Work out the finished part from the listing and answer in its coordinate system (mm). Face numbers are marked on the shaded views. Coordinates: 2 decimals unless noted, no trailing zeros. Write each loop counter-clockwise with the first axis right and the second up, starting at its lowest first coordinate (ties: lowest second). Pieces come first, ordered by that corner, then holes. Notation, with made-up numbers: (-38, 69.25) - (-27, 69.25) arc R34 cw to (-27, 101.25) - close; hole circle Ø8 at (11, 52). An arc over 180 degrees is marked (long way). Use CSV: the item, a comma, the result in double quotes. Start each with the question number.
from build123d import *

# Parameters (mm, degrees)
SKETCH1_W             = 48.6918
SKETCH1_H             = 39.1668
SKETCH1_R             = 4.7625
SKETCH1_R_2           = 3.175
BOSS_EXTRUDE1_DEPTH   = 7.62
CHAMFER1_SIZE         = 3.175
SKETCH3_W             = 39.1668
SKETCH3_H             = 29.6418
CUT_EXTRUDE2_DEPTH    = 1.27
F_4_CLEARANCE_HOLE1_D = 3.048
SKETCH7_R             = 4.415840843
SKETCH7_R_2           = 3.175
SKETCH7_R_3           = 1.5875
BOSS_EXTRUDE2_DEPTH   = 1.27
SKETCH15_R            = 6.0325
BOSS_EXTRUDE7_DEPTH   = 7.62
FILLET3_R             = 6.985
FILLET4_R             = 0.508


with BuildPart() as part:
    # Sketch1 → Boss-Extrude1 (new body)
    with BuildSketch(Plane.YZ):
        with Locations((-3.96875, 0)):
            Rectangle(SKETCH1_W, SKETCH1_H)
        with Locations(Location((-8.73125, 0, 0), (0, 0, 90))):
            Circle(SKETCH1_R, mode=Mode.SUBTRACT)
        with Locations(Location((8.73125, 0, 0), (0, 0, 90))):
            Circle(SKETCH1_R_2, mode=Mode.SUBTRACT)
    extrude(amount=BOSS_EXTRUDE1_DEPTH)

    # Chamfer1
    chamfer1_edges = [part.edges().sort_by_distance(p)[0] for p in [
        (3.81, 20.37715, -19.5834),
        (3.81, -28.31465, -19.5834),
        (3.81, -28.31465, 19.5834),
        (3.81, 20.37715, 19.5834),
    ]]
    chamfer(chamfer1_edges, length=CHAMFER1_SIZE)

    # Sketch3 → Cut-Extrude2 (cut)
    with BuildSketch(Plane(origin=(0, 0, 0), x_dir=(0, -1, 0), z_dir=(-1, 0, 0))):
        Polygon((-18.254252448, -22.1234), (26.191752448, -22.1234), (30.85465, -17.460502448), (30.85465, 17.460502448), (26.191752448, 22.1234), (-18.254252448, 22.1234), (-22.91715, 17.460502448), (-22.91715, -17.460502448), align=None)
        with Locations((3.96875, 0)):
            Rectangle(SKETCH3_W, SKETCH3_H, mode=Mode.SUBTRACT)
    extrude(amount=-CUT_EXTRUDE2_DEPTH, mode=Mode.SUBTRACT)

    # #4 Clearance Hole1 (through all)
    with Locations(Plane(origin=(1.27, 0, 0), x_dir=(0, -1, 0), z_dir=(-1, 0, 0))):
        with Locations((-17.9959, 9.525), (-11.90625, 17.20215), (3.96875, 17.20215), (19.84375, 17.20215), (25.9334, 9.525), (25.9334, -9.525), (19.84375, -17.20215), (3.96875, -17.20215), (-11.90625, -17.20215), (-17.9959, -9.525)):
            Hole(F_4_CLEARANCE_HOLE1_D / 2)

    # Sketch7 → Boss-Extrude2 (add)
    # profile 1 of 2: a face of its own
    with BuildSketch(Plane(origin=(0, 0, 0), x_dir=(0, -1, 0), z_dir=(-1, 0, 0))):
        with Locations((-8.73125, 0)):
            Circle(SKETCH7_R)
        with Locations(Location((-8.73125, 0, 0), (0, 0, 90))):
            Circle(SKETCH7_R_2, mode=Mode.SUBTRACT)
    # profile 2 of 2: a face of its own
    with BuildSketch(Plane(origin=(0, 0, 0), x_dir=(0, -1, 0), z_dir=(-1, 0, 0))):
        with Locations(Location((-8.73125, 0, 0), (0, 0, 90))):
            Circle(SKETCH7_R_2)
        with Locations(Location((-8.73125, 0, 0), (0, 0, 90))):
            Circle(SKETCH7_R_3, mode=Mode.SUBTRACT)
    extrude(amount=-BOSS_EXTRUDE2_DEPTH)

    # Sketch15 → Boss-Extrude7 (add)
    with BuildSketch(Plane.YZ.offset(7.62)):
        with Locations((-8.73125, 0)):
            Circle(SKETCH15_R)
    extrude(amount=-BOSS_EXTRUDE7_DEPTH)

    # Fillet3
    fillet3_edges = [part.edges().sort_by_distance(p)[0] for p in [
        (0.635, 15.61465, 14.8209),
        (0.635, -23.55215, 14.8209),
        (0.635, -23.55215, -14.8209),
        (0.635, 15.61465, -14.8209),
    ]]
    fillet(fillet3_edges, radius=FILLET3_R)

    # Fillet4
    fillet4_edges = [part.edges().sort_by_distance(p)[0] for p in [
        (4.445, -25.13965, -19.5834),
        (4.445, -28.31465, 16.4084),
        (4.445, 20.37715, -16.4084),
        (4.445, 17.20215, 19.5834),
        (4.445, -25.13965, 19.5834),
        (4.445, 20.37715, 16.4084),
        (4.445, 17.20215, -19.5834),
        (4.445, -28.31465, -16.4084),
    ]]
    fillet(fillet4_edges, radius=FILLET4_R)


solid = part.part
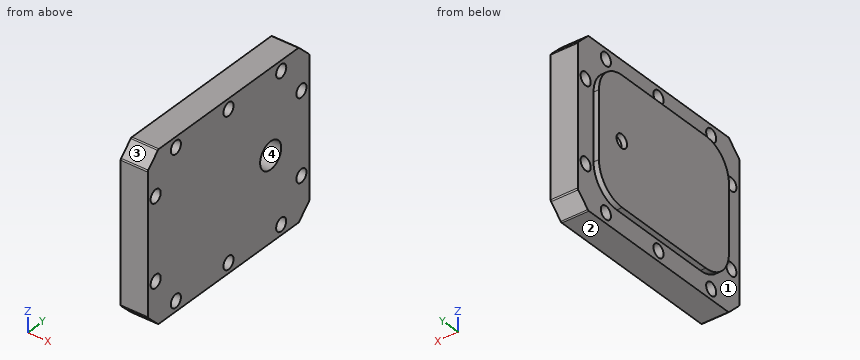
Item 1: Determine the mould class of the marked faces 1, 2, 3 and 4 for opening direction Z: +Z half, -Z half, draft (parallel to the pull), parting line (faces both ways), or undercut.
Item 2: Straight lines are drawn through the part: probe 1 along Z at (x, y) = (4.75, -20); probe 2 along Y at (x, z) = (3.5, 0); probe 3 along Z at (x, y) = (6, 8.5). For each, find the intervals that lie inside material, in ascending order. Write a range as [from, to].
Item 3: Each of these flat-tipped pins is pushed along its axis until it touches: pin 1 (2.5 mm diameter, centred on y = -19.84, z = 17.2, fed in from -X); pin 2 (0.6 mm diameter, centred on x = 0.5, z = 3, fed in from -Y); pin 3 (4 mm diameter, centred on y = 8.73, z = 0, fed in from +X); pin 4 (5 mm diameter, centred on y = 18, z = 9.52, fed in from -X). Where does it stop, or does it pass through?
Item 4: A cutting plane is placed at A-A (z = 0). Determine the outline of the cut face in (x, y), then the cut area to 3 significant figures.
Item 5: A cutting plane is placed at B-B (z = -6.5). Determine the outline of the cut face in (x, y), then the cut area to 3 significant figures.
Item 6: A cutting plane is placed at C-C (y = -9). Determine the outline of the cut face in (x, z), then the cut area to 3 significant figures.
Item 7: A cutting plane is placed at D-D (x = 3.5). Count the separate pieces of the cut face and the enclosed holes in it, then the cut area to 3 significant figures.
Calculated:
1,face 1,"draft"
1,face 2,"-Z half"
1,face 3,"+Z half"
1,face 4,"undercut"
2,probe 1,"z = [-19.58, -18.72], [-15.69, 15.69], [18.72, 19.58]"
2,probe 2,"y = [-28.31, 5.56], [11.91, 20.38]"
2,probe 3,"z = [-19.58, -3.17], [3.17, 19.58]"
3,pin 1,"passes through"
3,pin 2,"stops at y = -23.55"
3,pin 3,"stops at x = 1.27"
3,pin 4,"stops at x = 1.27"
4,outline,"(0, -23.55) - (1.27, -23.55) - (1.27, -28.31) - (7.62, -28.31) - (7.62, 5.56) - (1.27, 5.56) - (1.27, 7.14) - (0, 7.14) - close; (0, 10.32) - (1.27, 10.32) - (1.27, 11.91) - (7.62, 11.91) - (7.62, 20.38) - (1.27, 20.38) - (1.27, 15.61) - (0, 15.61) - close"
4,area,"315 mm²"
5,outline,"(0, -23.55) - (1.27, -23.55) - (1.27, -28.31) - (7.62, -28.31) - (7.62, 20.38) - (1.27, 20.38) - (1.27, 15.61) - (0, 15.61) - close"
5,area,"359 mm²"
6,outline,"(0, -14.82) - (1.27, -14.82) - (1.27, -19.58) - (7.62, -19.58) - (7.62, 19.58) - (1.27, 19.58) - (1.27, 14.82) - (0, 14.82) - close"
6,area,"286 mm²"
7,separate pieces,"1"
7,enclosed holes,"11"
7,area,"1,780 mm²"
